Part model, mm, in its own coordinate system. Give positions to 0.01 mm unless a question says otherwise; leave off trailing zeros. Write each loop counter-clockwise with the first axis right and the second up, starting at its lowest first coordinate (ties: lowest second). Pieces come first, ordered by that corner, then holes. Notation, with made-up numbers: M 81.5,-16 L 94.5,-16 A37 cw 94.5,22 Z; hole C -6.5,15 d10. An arc over 180 degrees is marked long. Use a Markdown table: item, result.
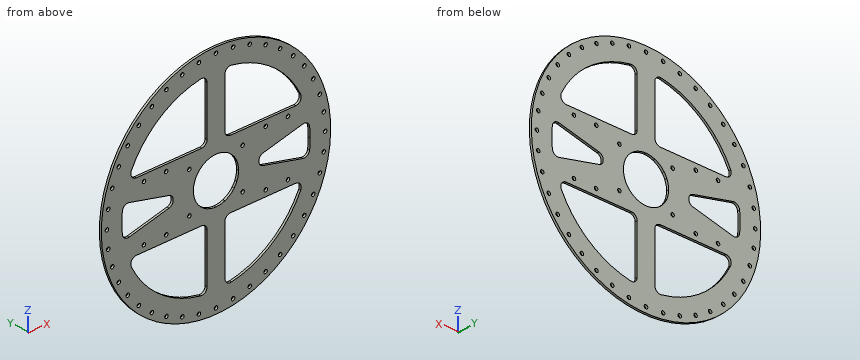
```python
from build123d import *

# Parameters (mm, degrees)
SKETCH_1_R          = 103.5
SKETCH_1_R_2        = 1.6
EXTRUDE_1_DEPTH     = 2
SKETCH_2_R          = 1.6
CUT_EXTRUDE_1_DEPTH = 147.384766967
SKETCH_3_W          = 8
SKETCH_3_H          = 8
CUT_EXTRUDE_2_DEPTH = 10
CUT_EXTRUDE_START   = -10
CUT_EXTRUDE_3_DEPTH = 10
FILLET_1_R          = 5


with BuildPart() as part:
    # 草图1 → 凸台-拉伸1 (new body)
    with BuildSketch(Plane(origin=(0, 0, 0), x_dir=(1, 0, 0), z_dir=(0, 1, 0))):
        with Locations(Location((0, 0, 0), (0, 0, 270))):
            Circle(SKETCH_1_R)
        with Locations(Location((-24, -18, 0), (0, 0, 270))):
            Circle(SKETCH_1_R_2, mode=Mode.SUBTRACT)
        with Locations(Location((24, -18, 0), (0, 0, 270))):
            Circle(SKETCH_1_R_2, mode=Mode.SUBTRACT)
        with Locations(Location((24, 18, 0), (0, 0, 270))):
            Circle(SKETCH_1_R_2, mode=Mode.SUBTRACT)
        with Locations(Location((-24, 18, 0), (0, 0, 270))):
            Circle(SKETCH_1_R_2, mode=Mode.SUBTRACT)
    extrude(amount=EXTRUDE_1_DEPTH)

    # 草图2 → 切除-拉伸1 (cut, through all)
    with BuildSketch(Plane(origin=(0, 2, 0), x_dir=(1, 0, 0), z_dir=(0, 1, 0))):
        with Locations(Location((-45, 24.5, 0), (0, 0, 270))):
            Circle(SKETCH_2_R)
        with Locations(Location((-65, 24.5, 0), (0, 0, 270))):
            Circle(SKETCH_2_R)
        with Locations(Location((-65, -24.5, 0), (0, 0, 270))):
            Circle(SKETCH_2_R)
        with Locations(Location((-45, -24.5, 0), (0, 0, 270))):
            Circle(SKETCH_2_R)
        with Locations(Location((45, -24.5, 0), (0, 0, 270))):
            Circle(SKETCH_2_R)
        with Locations(Location((65, -24.5, 0), (0, 0, 270))):
            Circle(SKETCH_2_R)
        with Locations(Location((45, 24.5, 0), (0, 0, 270))):
            Circle(SKETCH_2_R)
        with Locations(Location((65, 24.5, 0), (0, 0, 270))):
            Circle(SKETCH_2_R)
        with Locations(Location((0, 98.5, 0), (0, 0, 270))):
            Circle(SKETCH_2_R)
        with Locations(Location((15.408794806, 97.287301549, 0), (0, 0, 270))):
            Circle(SKETCH_2_R)
        with Locations(Location((30.438173946, 93.679066855, 0), (0, 0, 270))):
            Circle(SKETCH_2_R)
        with Locations(Location((44.718064224, 87.764142633, 0), (0, 0, 270))):
            Circle(SKETCH_2_R)
        with Locations(Location((57.896847351, 79.688173946, 0), (0, 0, 270))):
            Circle(SKETCH_2_R)
        with Locations(Location((69.650017947, 69.650017947, 0), (0, 0, 270))):
            Circle(SKETCH_2_R)
        with Locations(Location((79.688173946, 57.896847351, 0), (0, 0, 270))):
            Circle(SKETCH_2_R)
        with Locations(Location((87.764142633, 44.718064224, 0), (0, 0, 270))):
            Circle(SKETCH_2_R)
        with Locations(Location((93.679066855, 30.438173946, 0), (0, 0, 270))):
            Circle(SKETCH_2_R)
        with Locations(Location((97.287301549, 15.408794806, 0), (0, 0, 270))):
            Circle(SKETCH_2_R)
        with Locations(Location((98.5, 0, 0), (0, 0, 270))):
            Circle(SKETCH_2_R)
        with Locations(Location((97.287301549, -15.408794806, 0), (0, 0, 270))):
            Circle(SKETCH_2_R)
        with Locations(Location((93.679066855, -30.438173946, 0), (0, 0, 270))):
            Circle(SKETCH_2_R)
        with Locations(Location((87.764142633, -44.718064224, 0), (0, 0, 270))):
            Circle(SKETCH_2_R)
        with Locations(Location((79.688173946, -57.896847351, 0), (0, 0, 270))):
            Circle(SKETCH_2_R)
        with Locations(Location((69.650017947, -69.650017947, 0), (0, 0, 270))):
            Circle(SKETCH_2_R)
        with Locations(Location((57.896847351, -79.688173946, 0), (0, 0, 270))):
            Circle(SKETCH_2_R)
        with Locations(Location((44.718064224, -87.764142633, 0), (0, 0, 270))):
            Circle(SKETCH_2_R)
        with Locations(Location((30.438173946, -93.679066855, 0), (0, 0, 270))):
            Circle(SKETCH_2_R)
        with Locations(Location((15.408794806, -97.287301549, 0), (0, 0, 270))):
            Circle(SKETCH_2_R)
        with Locations(Location((0, -98.5, 0), (0, 0, 270))):
            Circle(SKETCH_2_R)
        with Locations(Location((-15.408794806, -97.287301549, 0), (0, 0, 270))):
            Circle(SKETCH_2_R)
        with Locations(Location((-30.438173946, -93.679066855, 0), (0, 0, 270))):
            Circle(SKETCH_2_R)
        with Locations(Location((-44.718064224, -87.764142633, 0), (0, 0, 270))):
            Circle(SKETCH_2_R)
        with Locations(Location((-57.896847351, -79.688173946, 0), (0, 0, 270))):
            Circle(SKETCH_2_R)
        with Locations(Location((-69.650017947, -69.650017947, 0), (0, 0, 270))):
            Circle(SKETCH_2_R)
        with Locations(Location((-79.688173946, -57.896847351, 0), (0, 0, 270))):
            Circle(SKETCH_2_R)
        with Locations(Location((-87.764142633, -44.718064224, 0), (0, 0, 270))):
            Circle(SKETCH_2_R)
        with Locations(Location((-93.679066855, -30.438173946, 0), (0, 0, 270))):
            Circle(SKETCH_2_R)
        with Locations(Location((-97.287301549, -15.408794806, 0), (0, 0, 270))):
            Circle(SKETCH_2_R)
        with Locations(Location((-98.5, 0, 0), (0, 0, 270))):
            Circle(SKETCH_2_R)
        with Locations(Location((-97.287301549, 15.408794806, 0), (0, 0, 270))):
            Circle(SKETCH_2_R)
        with Locations(Location((-93.679066855, 30.438173946, 0), (0, 0, 270))):
            Circle(SKETCH_2_R)
        with Locations(Location((-87.764142633, 44.718064224, 0), (0, 0, 270))):
            Circle(SKETCH_2_R)
        with Locations(Location((-79.688173946, 57.896847351, 0), (0, 0, 270))):
            Circle(SKETCH_2_R)
        with Locations(Location((-69.650017947, 69.650017947, 0), (0, 0, 270))):
            Circle(SKETCH_2_R)
        with Locations(Location((-57.896847351, 79.688173946, 0), (0, 0, 270))):
            Circle(SKETCH_2_R)
        with Locations(Location((-44.718064224, 87.764142633, 0), (0, 0, 270))):
            Circle(SKETCH_2_R)
        with Locations(Location((-30.438173946, 93.679066855, 0), (0, 0, 270))):
            Circle(SKETCH_2_R)
        with Locations(Location((-15.408794806, 97.287301549, 0), (0, 0, 270))):
            Circle(SKETCH_2_R)
    extrude(amount=-CUT_EXTRUDE_1_DEPTH, mode=Mode.SUBTRACT)

    # 草图3 → 切除-拉伸2 (cut)
    with BuildSketch(Plane(origin=(0, 2, 0), x_dir=(1, 0, 0), z_dir=(0, 1, 0))):
        with BuildLine():
            ThreePointArc((-79.529868603, -30), (-51.587586632, -67.555317374), (-8, -84.622691992))
            Line((-8, -84.622691992), (-8, -30))
            Line((-8, -30), (-79.529868603, -30))
        make_face()
        with BuildLine():
            Line((8, -30), (8, -84.622691992))
            ThreePointArc((8, -84.622691992), (51.587586632, -67.555317374), (79.529868603, -30))
            Line((79.529868603, -30), (8, -30))
        make_face()
        with BuildLine():
            Line((8, 30), (79.529868603, 30))
            ThreePointArc((79.529868603, 30), (51.587586632, 67.555317374), (8, 84.622691992))
            Line((8, 84.622691992), (8, 30))
        make_face()
        with BuildLine():
            ThreePointArc((-8, 84.622691992), (-51.587586632, 67.555317374), (-79.529868603, 30))
            Line((-79.529868603, 30), (-8, 30))
            Line((-8, 30), (-8, 84.622691992))
        make_face()
        with BuildLine():
            Line((-18.765926569, 8), (-8, 8))
            Line((-8, 8), (-8, 18.765926569))
            ThreePointArc((-8, 18.765926569), (-12.590175955, 16.051400856), (-16.320000071, 12.239999905))
            ThreePointArc((-16.320000071, 12.239999905), (-17.670595968, 10.19362733), (-18.765926569, 8))
        make_face()
        with BuildLine():
            Line((-20.4, 0), (-8, 0))
            Line((-8, 0), (-8, 8))
            Line((-8, 8), (-18.765926569, 8))
            ThreePointArc((-18.765926569, 8), (-19.987307247, 4.082590966), (-20.4, 0))
        make_face()
        with BuildLine():
            Line((-18.765926569, -8), (-8, -8))
            Line((-8, -8), (-8, 0))
            Line((-8, 0), (-20.4, 0))
            ThreePointArc((-20.4, 0), (-19.987307247, -4.082590966), (-18.765926569, -8))
        make_face()
        with BuildLine():
            ThreePointArc((-16.320000071, -12.239999905), (-12.590175955, -16.051400856), (-8, -18.765926569))
            Line((-8, -18.765926569), (-8, -8))
            Line((-8, -8), (-18.765926569, -8))
            ThreePointArc((-18.765926569, -8), (-17.670595968, -10.19362733), (-16.320000071, -12.239999905))
        make_face()
        with BuildLine():
            ThreePointArc((-8, -18.765926569), (-4.082590966, -19.987307247), (0, -20.4))
            Line((0, -20.4), (0, -8))
            Line((0, -8), (-8, -8))
            Line((-8, -8), (-8, -18.765926569))
        make_face()
        with BuildLine():
            Line((0, -8), (0, -20.4))
            ThreePointArc((0, -20.4), (4.082590966, -19.987307247), (8, -18.765926569))
            Line((8, -18.765926569), (8, -8))
            Line((8, -8), (0, -8))
        make_face()
        with Locations((4, -4)):
            Rectangle(SKETCH_3_W, SKETCH_3_H)
        with Locations((-4, -4)):
            Rectangle(SKETCH_3_W, SKETCH_3_H)
        with Locations((-4, 4)):
            Rectangle(SKETCH_3_W, SKETCH_3_H)
        with Locations((4, 4)):
            Rectangle(SKETCH_3_W, SKETCH_3_H)
        with BuildLine():
            Line((0, 20.4), (0, 8))
            Line((0, 8), (8, 8))
            Line((8, 8), (8, 18.765926569))
            ThreePointArc((8, 18.765926569), (4.082590966, 19.987307247), (0, 20.4))
        make_face()
        with BuildLine():
            Line((-8, 8), (0, 8))
            Line((0, 8), (0, 20.4))
            ThreePointArc((0, 20.4), (-4.082590966, 19.987307247), (-8, 18.765926569))
            Line((-8, 18.765926569), (-8, 8))
        make_face()
        with BuildLine():
            Line((8, 18.765926569), (8, 8))
            Line((8, 8), (18.765926569, 8))
            ThreePointArc((18.765926569, 8), (17.670595876, 10.193627488), (16.319999852, 12.240000197))
            ThreePointArc((16.319999852, 12.240000197), (12.590175811, 16.051400968), (8, 18.765926569))
        make_face()
        with BuildLine():
            Line((8, 8), (8, 0))
            Line((8, 0), (20.4, 0))
            ThreePointArc((20.4, 0), (19.987307247, 4.082590966), (18.765926569, 8))
            Line((18.765926569, 8), (8, 8))
        make_face()
        with BuildLine():
            Line((8, 0), (8, -8))
            Line((8, -8), (18.765926569, -8))
            ThreePointArc((18.765926569, -8), (19.987307247, -4.082590966), (20.4, 0))
            Line((20.4, 0), (8, 0))
        make_face()
        with BuildLine():
            Line((8, -8), (8, -18.765926569))
            ThreePointArc((8, -18.765926569), (12.59017607, -16.051400765), (16.320000248, -12.23999967))
            ThreePointArc((16.320000248, -12.23999967), (17.670596041, -10.193627203), (18.765926569, -8))
            Line((18.765926569, -8), (8, -8))
        make_face()
    extrude(amount=-CUT_EXTRUDE_2_DEPTH, mode=Mode.SUBTRACT)

    # 草图4 → 切除-拉伸3 (cut)
    with BuildSketch(Plane.XZ.offset(CUT_EXTRUDE_START)):
        with BuildLine():
            ThreePointArc((-83.7368024, 14.599586429), (-85, 0), (-83.7368024, -14.599586429))
            Line((-83.7368024, -14.599586429), (-21.794871795, 0))
            Line((-21.794871795, 0), (-83.7368024, 14.599586429))
        make_face()
        with BuildLine():
            Line((83.7368024, 14.599586429), (21.794871795, 0))
            Line((21.794871795, 0), (83.7368024, -14.599586429))
            ThreePointArc((83.7368024, -14.599586429), (84.683611767, -7.327066126), (85, 0))
            ThreePointArc((85, 0), (84.683611767, 7.327066126), (83.7368024, 14.599586429))
        make_face()
    extrude(amount=CUT_EXTRUDE_3_DEPTH, mode=Mode.SUBTRACT)

    # 圆角1
    fillet_1_edges = [part.edges().sort_by_distance(p)[0] for p in [
        (8, 1, 84.622691992),
        (8, 1, 30),
        (79.529868603, 1, 30),
        (79.529868603, 1, -30),
        (8, 1, -30),
        (8, 1, -84.622691992),
        (-8, 1, -84.622691992),
        (-8, 1, -30),
        (-79.529868603, 1, -30),
        (-79.529868603, 1, 30),
        (-8, 1, 30),
        (-8, 1, 84.622691992),
        (-83.7368024, 1, 14.599586429),
        (-21.794871795, 1, 0),
        (-83.7368024, 1, -14.599586429),
        (83.7368024, 1, -14.599586429),
        (21.794871795, 1, 0),
        (83.7368024, 1, 14.599586429),
    ]]
    fillet(fillet_1_edges, radius=FILLET_1_R)


solid = part.part
```
1. Cut at A-A, the plane x = -51. Give the cut face in (y, z), then the cut area to 3 significant figures.
Findings below:
| item | result |
|---|---|
| outline | M 0,-90.06 L 2,-90.06 L 2,-68 L 0,-68 Z; M 0,-30 L 2,-30 L 2,-6.88 L 0,-6.88 Z; M 0,6.88 L 2,6.88 L 2,30 L 0,30 Z; M 0,68 L 2,68 L 2,90.06 L 0,90.06 Z |
| area | 181 mm2 |
2. Drop flat-ended pins along their axis: P1, Ø1, axis at x = 61, z = 70.5, coming from the -Y side; P2, Ø2.5, axis at x = 98.5, z = 0, coming from the -Y side; P3, Ø0.6, axis at y = 0.5, z = 57.5, coming from the +X side; P4, Ø0.6, axis at x = -30, y = 1, coming from the -Z side. Give the stop position or say it passes through.
Findings below:
| item | result |
|---|---|
| P1 | y = 0 |
| P2 | through |
| P3 | x = 86.26 |
| P4 | z = -99.15 |
3. Cut at B-B, the plane y = 1.55. State how many separate pieces and enclosed holes the cut face has, then the cut area to 3 significant figures.
Findings below:
| item | result |
|---|---|
| separate pieces | 1 |
| enclosed holes | 59 |
| area | 19,400 mm2 |
4. Drill centre lines: L1, parallel to X at y = 0.95, z = 39; L2, parallel to Z at x = -72.5, y = 0.95; L3, parallel to Z at x = 33.5, y = 1.5. Where is each one in solid material? Low to high.
Findings below:
| item | result |
|---|---|
| L1 | -95.87 to -75.52, -8 to 8, 75.52 to 95.87 |
| L2 | -73.86 to -44.37, -30.03 to -11.95, 11.95 to 30.03, 44.37 to 73.86 |
| L3 | -97.93 to -78.12, -30 to 30, 78.12 to 97.93 |
